```python
from build123d import *

# Parameters (mm, degrees)
F1_DEPTH = 63.5
F2_DEPTH = 25.4
F3_DEPTH = 7.9375
F0_W     = 25.4
F0_H     = 4.7752
F5_R     = 6.35


with BuildPart() as f1:
    # F0 (on Front) → F1 (new body, symmetric)
    with BuildSketch(Plane.XZ):
        Polygon((22.225, 9.525), (-41.275, 9.525), (-41.275, -9.525), (41.275, -9.525), (41.275, 9.525), align=None)
    extrude(amount=F1_DEPTH, both=True)

    # F0 (on Front) → F2 (join, symmetric)
    with BuildSketch(Plane.XZ):
        with BuildLine():
            Line((22.225, 27.0002), (22.225, 9.525))
            Line((22.225, 9.525), (41.275, 9.525))
            Line((41.275, 9.525), (41.275, 27.0002))
            ThreePointArc((41.275, 27.0002), (45.9246798487, 38.2255201513), (57.15, 42.8752))
            Line((57.15, 42.8752), (60.325, 42.8752))
            Line((60.325, 42.8752), (60.325, 61.9476745522))
            Line((60.325, 61.9476745522), (57.15, 61.9252))
            ThreePointArc((57.15, 61.9252), (32.4542956671, 51.6959043329), (22.225, 27.0002))
        make_face()
        Polygon((85.725, 62.1274709702), (60.325, 61.9476745522), (60.325, 42.8752), (85.725, 42.8752), align=None)
    extrude(amount=F2_DEPTH, both=True)

    # F0 (on Front) → F3 (join, symmetric)
    with BuildSketch(Plane.XZ):
        with BuildLine():
            add(Edge.make_bspline(
                [(-41.275, 9.525), (-12.9327131435, 46.9444841146), (11.8099329993, 63.8144686818), (57.15, 61.9252)],
                knots=[0, 0, 0, 0, 111.5045361635, 111.5045361635, 111.5045361635, 111.5045361635], degree=3))
            Line((-41.275, 9.525), (22.225, 9.525))
            Line((22.225, 9.525), (22.225, 27.0002))
            ThreePointArc((22.225, 27.0002), (32.4542956671, 51.6959043329), (57.15, 61.9252))
        make_face()
    extrude(amount=F3_DEPTH, both=True)

    # F0 (on Front) → F4 (revolve)
    with BuildSketch(Plane.XZ):
        Polygon((85.725, 66.675), (85.725, 62.1274709702), (85.725, 42.8752), (111.125, 42.8752), (111.125, 66.675), align=None)
        with Locations((98.425, 40.4876)):
            Rectangle(F0_W, F0_H)
    revolve(axis=Axis((85.725, 0, 52.3875), (0, 0, 1)))

    # F5
    f5_edges = [f1.edges().sort_by_distance(p)[0] for p in [
        (-41.275, -63.5, 0),
        (41.275, -63.5, 0),
        (41.275, 63.5, 0),
        (-41.275, 63.5, 0),
    ]]
    fillet(f5_edges, radius=F5_R)


solid = f1.part
```
Source: CAD feature listing. Evaluate the final solid. Frame: model axes, mm. A direction names the side the tool comes from. Give positions to 0.01 mm unless a question says otherwise; leave off trailing zeros. Loops run counter-clockwise (first coordinate to the right, second up) from the corner with the lowest first, then second, coordinate; pieces in that order, holes last. Notation, with made-up numbers: M 2.25,37.25 L 59.25,37.25 A10 cw 59.25,48.25 Z; hole C 37,13.5 d11. An arc over 180 degrees is marked long. Put each result on its own line as item: value.
Q1. Line query: probe 1 along Z at (x, y) = (-29.5, 24) (3 decimals); probe 2 along Y at (x, z) = (40, 56); probe 3 along Y at (x, z) = (-13, 39.5). Output: solid intervals per line, ascending. Write a range as [from, to].
Response values:
probe 1: z = [-9.525, 9.525]
probe 2: y = [-25.4, 25.4]
probe 3: y = [-7.94, 7.94]
Q2. Section C-C (y = 51.5). Return the cut outline in (x, z) (3 decimals), and give its area (3 significant figures).
Response values:
outline: M -41.275,-9.525 L 41.275,-9.525 L 41.275,9.525 L -41.275,9.525 Z
area: 1,570 mm²
Q3. Section A-A (z = 7.5). Return the cut outline in (x, y) (3 decimals).
Response values:
outline: M -41.275,-57.15 A6.35 ccw -34.925,-63.5 L 34.925,-63.5 A6.35 ccw 41.275,-57.15 L 41.275,57.15 A6.35 ccw 34.925,63.5 L -34.925,63.5 A6.35 ccw -41.275,57.15 Z
Q4. Reachability of faces 5 (the flat face through (86, 0, 38.1)), 6 (the cylindrical face through (32.73, 16.55, 51.97)), 7 (the flat face through (46, 25.4, 42)), 8 (the flat face through (22.225, -17, 18)), 9 (the cylindrical face through (39.464, -61.59, 0.133)) from +Z, -Z, +X, -X, +Y, -Y: full face, straight path, thin tool, end or side. Return the list, or none.
Response values:
face 5: -Z, +X, +Y, -Y
face 6: +Z, -X, +Y
face 7: +Z, +X, -X, +Y
face 8: +Z, -X, -Y
face 9: +Z, -Z, +X, -Y
Q5. Pin query (flat end, axial travel): P1, Ø1, axis at x = -5, y = -29, coming from the +Z side (3 decimals); P2, Ø19, axis at y = -18, z = 22.5, coming from the -X side (3 decimals); P3, Ø4, axis at x = -15, z = 25.5, coming from the -Y side. Return the tip coordinate at first contact, or that it passes through.
Response values:
P1: stops at z = 9.525
P2: stops at x = 22.225
P3: stops at y = -7.94
Q6. Section B-B (x = 72). Return the cut outline in (y, z) (3 decimals), and give its area (3 significant figures).
Response values:
outline: M -25.4,42.875 L -21.373,42.875 L -21.373,38.1 L 21.373,38.1 L 21.373,42.875 L 25.4,42.875 L 25.4,62.03 L 21.373,62.03 L 21.373,66.675 L -21.373,66.675 L -21.373,62.03 L -25.4,62.03 Z
area: 1,380 mm²
Q7. Mould query, pull axis X, two halves, no side actions, for faces 1 (the cylindrical face through (39.464, 61.59, 0.133)), 2 (the flat face through (1, -36, 9.525)), 3 (the cylindrical face through (45.8, -0.4, 38.1)), 4 (the cylindrical face through (32.73, -16.79, 51.97)). Classes: released by +X, released by -X, zero draft, split by the parting line, or undercut.
Response values:
face 1: released by +X
face 2: zero draft
face 3: undercut
face 4: released by -X
